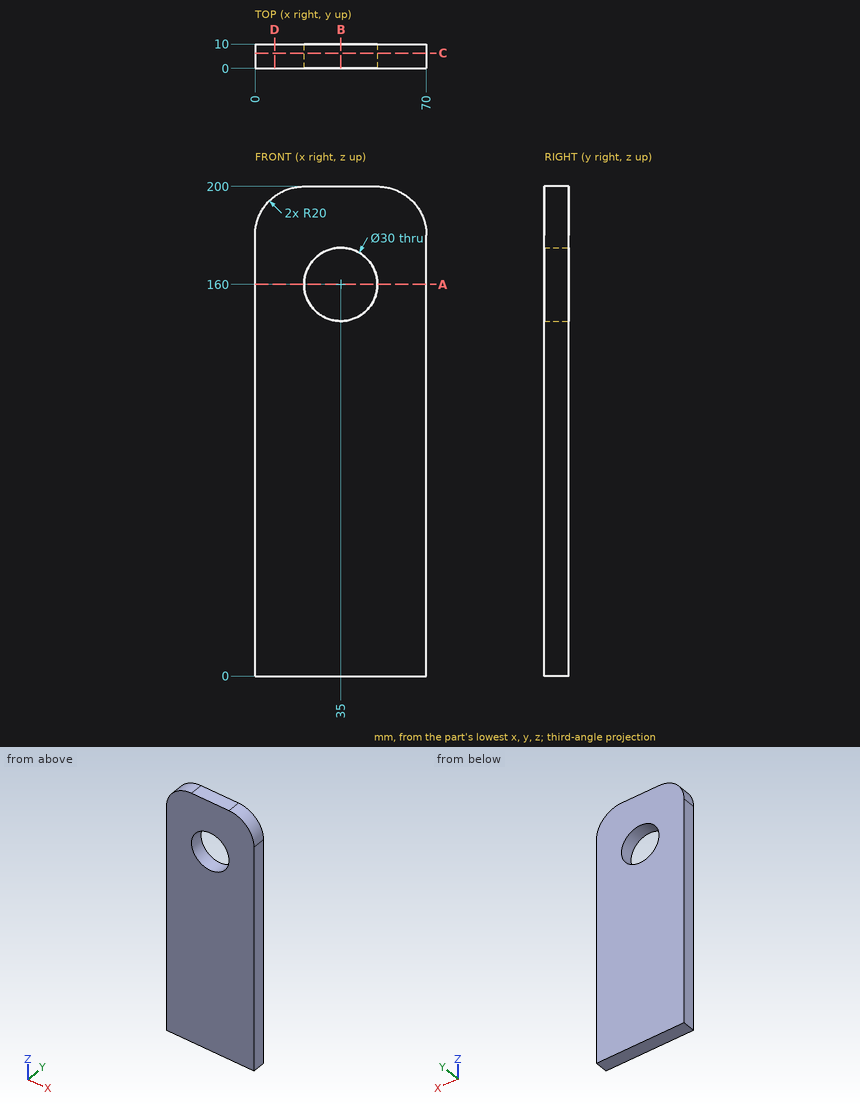
Part print with two shaded views. Sizes in mm from the minimum x, y, z corner. Give positions to 0.01 mm unless a question says otherwise; leave off trailing zeros. Order: outer loops, then holes, each group sorted by start corner. A loop starts at its lowest first (then second) coordinate and runs counter-clockwise, first axis right, second up.
1) Pin check, flat tips, straight feed: pin 1 (5 mm diameter, centred on x = 55, y = 2.5, fed in from +Z); pin 2 (1 mm diameter, centred on x = 22.5, z = 42.5, fed in from -Y); pin 3 (1 mm diameter, centred on x = 58.5, y = 8.5, fed in from +Z). Stop position of each tip, or through.
2) Wall check: probe 1 along Z at (x, y) = (35, 3.5); probe 2 along X at (y, z) = (2.25, 160); probe 3 along Z at (x, y) = (43, 4.5). Give the ranges that are in metal, low to high.
3) Saw through at A-A, the plane z = 160. Write the cut outline in (x, y).
4) Saw through at C-C, the plane y = 6.25. Write the cut outline in (x, z), then the cut area to 3 significant figures.
5) Saw through at B-B, the plane x = 35. Write the cut outline in (y, z).
6) Saw through at D-D, the plane x = 8. Write the cut outline in (y, z), then the cut area to 3 significant figures.
Computed:
1. pin 1: stops at z = 199.84
1. pin 2: stops at y = 0
1. pin 3: stops at z = 198.33
2. probe 1: z = 0 to 145, 175 to 200
2. probe 2: x = 0 to 20, 50 to 70
2. probe 3: z = 0 to 147.31, 172.69 to 200
3. outline: (0, 0) - (20, 0) - (20, 10) - (0, 10) - close; (50, 0) - (70, 0) - (70, 10) - (50, 10) - close
4. outline: (0, 0) - (70, 0) - (70, 180) arc R20 ccw to (50, 200) - (20, 200) arc R20 ccw to (0, 180) - close; hole circle Ø30 at (35, 160)
4. area: 13,100 mm2
5. outline: (0, 0) - (10, 0) - (10, 145) - (0, 145) - close; (0, 175) - (10, 175) - (10, 200) - (0, 200) - close
6. outline: (0, 0) - (10, 0) - (10, 196) - (0, 196) - close
6. area: 1,960 mm2
